Read the model definition and answer for the solid it produces. Units are mm, in the model's axes. Round coordinates to 2 decimals unless told otherwise and drop trailing zeros. Order: outer loops, then holes, each group sorted by start corner. A loop starts at its lowest first (then second) coordinate and runs counter-clockwise, first axis right, second up. Notation, with made-up numbers: (82.5, 39.25) -> (108.5, 39.25) arc R21 ccw to (108.5, 45.25) -> close; hole circle Ø2 at (-24, 28.25). An arc over 180 degrees is marked (long way). Use a Markdown table: item, result. Add a question column.
1. Section A-A, the plane z = 130.5 is taken. Give the vertices of the cut face in (x, y) (1 decimal), then the cut area to 3 significant figures.
2. Section B-B, the plane y = 0 is taken. Give the number of separate pieces and of enclosed holes in the cut face, then the cut area to 3 significant figures.
3. Consider L1, parallel to X at y = -8.45, z = 76.2 (3 decimals); L2, parallel to X at y = -6, z = -126 (1 decimal). Determine where each line is inside the solid, lowest interval first. Write a range as [from, to].
4. Given pin 1 (1 mm diameter, centred on x = 4, y = -5.5, fed in from -Z), flat-ended and moving along its own axis, determine where the tip first touches the part or whether it passes through.
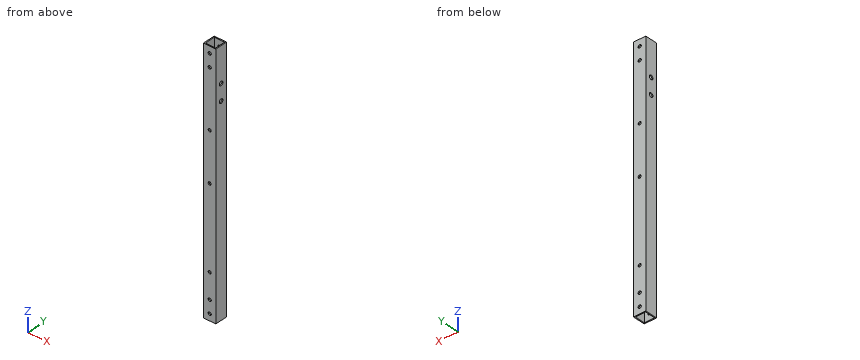
```python
from build123d import *

# Parameters (mm, degrees)
SKETCH1_W           = 19.05
SKETCH1_H           = 19.05
SKETCH1_W_2         = 15.875
SKETCH1_H_2         = 15.875
BOSS_EXTRUDE1_DEPTH = 196.85
SKETCH2_R           = 2.5
CUT_EXTRUDE1_DEPTH  = 30
SKETCH3_R           = 3.2639
CUT_EXTRUDE2_DEPTH  = 30
SKETCH4_R           = 2.38125
CUT_EXTRUDE3_DEPTH  = 30


with BuildPart() as part:
    # Sketch1 → Boss-Extrude1 (new, symmetric)
    with BuildSketch(Plane.XY):
        Rectangle(SKETCH1_W, SKETCH1_H)
        Rectangle(SKETCH1_W_2, SKETCH1_H_2, mode=Mode.SUBTRACT)
    extrude(amount=BOSS_EXTRUDE1_DEPTH, both=True)

    # Sketch2 → Cut-Extrude1 (cut)
    with BuildSketch(Plane(origin=(0, 13.525, 0), x_dir=(1, 0, 0), z_dir=(0, 1, 0))):
        with Locations(Location((0, -186.375, 0), (0, 0, 270))):
            Circle(SKETCH2_R)
        with Locations(Location((0, -166.375, 0), (0, 0, 270))):
            Circle(SKETCH2_R)
    cut_extrude1 = extrude(amount=-CUT_EXTRUDE1_DEPTH, mode=Mode.SUBTRACT)

    # Mirror1: Cut-Extrude1 across Front Plane
    add(cut_extrude1.mirror(Plane.XY), mode=Mode.SUBTRACT)

    # Sketch3 → Cut-Extrude2 (cut)
    with BuildSketch(Plane.ZY.offset(14.3002)):
        with Locations(Location((142.675, 0, 0), (0, 0, 180))):
            Circle(SKETCH3_R)
        with Locations(Location((117.275, 0, 0), (0, 0, 180))):
            Circle(SKETCH3_R)
    extrude(amount=-CUT_EXTRUDE2_DEPTH, mode=Mode.SUBTRACT)

    # Sketch4 → Cut-Extrude3 (cut)
    with BuildSketch(Plane(origin=(0, 18.1864, 0), x_dir=(1, 0, 0), z_dir=(0, 1, 0))):
        with Locations(Location((0, 0, 0), (0, 0, 270))):
            Circle(SKETCH4_R)
        with Locations(Location((0, 127, 0), (0, 0, 270))):
            Circle(SKETCH4_R)
        with Locations(Location((0, -76.2, 0), (0, 0, 270))):
            Circle(SKETCH4_R)
    extrude(amount=-CUT_EXTRUDE3_DEPTH, mode=Mode.SUBTRACT)


solid = part.part
```
Verdict:
| question | item | result |
|---|---|---|
| 1 | outline | (-9.5, -9.5) -> (9.5, -9.5) -> (9.5, 9.5) -> (-9.5, 9.5) -> close; hole (-7.9, -7.9) -> (7.9, -7.9) -> (7.9, 7.9) -> (-7.9, 7.9) -> close |
| 1 | area | 111 mm2 |
| 2 | separate pieces | 6 |
| 2 | enclosed holes | 0 |
| 2 | area | 1,210 mm2 |
| 3 | L1 | x = [-9.525, -2.381], [2.381, 9.525] |
| 3 | L2 | x = [-9.5, -7.9], [7.9, 9.5] |
| 4 | pin 1 | passes through |
